Source: CAD feature listing. Evaluate the final solid. Frame: model axes, mm. Give positions to 0.01 mm unless a question says otherwise; leave off trailing zeros. Write each loop counter-clockwise with the first axis right and the second up, starting at its lowest first coordinate (ties: lowest second). Pieces come first, ordered by that corner, then holes. Notation, with made-up numbers: (82.5, 43) - (113.5, 43) arc R23 cw to (113.5, 81) - close; hole circle Ø3 at (35.5, -29.75). An arc over 180 degrees is marked (long way). One line per question, with ' | ' between items. Start each with the question number.
(1) Section A-A, the plane z = 2.75. Return loops of the section in (x, y) (3 decimals).
(2) Section D-D, the plane y = 2.75. Return loops of the section in (x, z) (3 decimals), plus the area to 3 significant figures.
(3) Ray query, line 1 (Y direction, x = 1, z = 17.75) (3 decimals); line 2 (Z direction, x = 1.05, y = 14.25); line 3 (Y direction, x = 1.45, z = 2). Return the intervals inside material, ascending. Write a range as [from, to].
(4) Draft query along Z for faces 1 (the flat face through (1.6, 13, 10)), 2 (the cylindrical face through (0.81, 22.63, 16.25)), 3 (the flat face through (1, 13, 0)). Return one class per face: +Z half, -Z half, draft (parallel to the pull), parting line (faces both ways), or undercut.
(5) Section B-B, the plane x = 0.35. State how many separate pieces and enclosed holes the cut face has, plus the area to 3 significant figures.
Autodesk Inventor part; units mm, degrees
ref_plane "YZ Plane" through (0, 0, 0) normal (1, 0, 0) x (0, 1, 0)
ref_plane "XZ Plane" through (0, 0, 0) normal (0, 1, 0) x (-1, 0, 0)
ref_plane "XY Plane" through (0, 0, 0) normal (0, 0, 1) x (1, 0, 0)
sketch "Náčrt1" plane through (0, 0, 0) normal (1, 0, 0) x (0, 1, 0)
  line L0 (0, 0) -> (26, 0)
  line L1 (26, 0) -> (26, 20.3)
  line L2 (26, 20.3) -> (0, 20.3)
  line L3 (0, 20.3) -> (0, 0)
  dimension "d0" = 26
  dimension "d1" = 20.3
extrude "Vysunutí1" add sketch "Náčrt1" along normal blind 1.6
sketch "Náčrt2" plane through (1.6, 0, 0) normal (1, 0, 0) x (0, 0, -1)
  line L0 (0, 0) -> (0, 26)
  line L1 (-20.3, 0) -> (0, 0)
  circle A0 centre (-2.75, 23.25) radius 1.625
  circle A1 centre (-2.75, 2.75) radius 1.625
  circle A2 centre (-1.27, 16.81) radius 0.45
  circle A3 centre (-1.27, 14.27) radius 0.45
  circle A4 centre (-1.27, 11.73) radius 0.45
  circle A5 centre (-1.27, 9.19) radius 0.45
  circle A6 centre (-17.75, 23.25) radius 1.625
  circle A7 centre (-17.75, 2.75) radius 1.625
  dimension "d4" = 20.5
  dimension "d6" = 3.25
  dimension "d7" = 2.75
  dimension "d8" = 2.75
  dimension "d9" = 2.75
  dimension "d10" = 0.9
  dimension "d11" = 1.27
  dimension "d12" = 2.54
  dimension "d13" = 2.54
  dimension "d14" = 2.54
  dimension "d15" = 1.27
  dimension "d16" = 1.27
  dimension "d17" = 1.27
  dimension "d18" = 7.62
  dimension "d19" = 6.44
  dimension "d20" = 20.5
  dimension "d21" = 2.75
  dimension "d25" = 15
  dimension "d26" = 15
extrude "Vysunutí3" cut sketch "Náčrt2" against normal through all
sketch "Náčrt3" plane through (1.6, 0, 0) normal (1, 0, 0) x (0, 0, -1)
  circle A0 centre (-1.27, 11.73) radius 0.45
  circle A1 centre (-1.27, 16.81) radius 0.45
  circle A2 centre (-1.27, 14.27) radius 0.45
  circle A3 centre (-1.27, 9.19) radius 0.45
  line L0 (-2.27, 17.7223) -> (-0.27, 17.7223)
  line L1 (-0.27, 17.7223) -> (-0.27, 15.7223)
  line L2 (-0.27, 15.7223) -> (-2.27, 15.7223)
  line L3 (-2.27, 15.7223) -> (-2.27, 17.7223)
  circle A4 centre (-1.27, 14.27) radius 1
  circle A5 centre (-1.27, 11.73) radius 1
  circle A6 centre (-1.27, 9.19) radius 1
  dimension "d31" = 2
  dimension "d33" = 1
  dimension "d34" = 2
  dimension "d35" = 1.0877
  dimension "d36" = 2
extrude "Vysunutí4" add sketch "Náčrt3" along normal blind 0.001
sketch "Náčrt4" plane through (0, 0, 0) normal (-1, 0, 0) x (0, 0, 1)
  circle A0 centre (1.27, 11.73) radius 0.45
  circle A1 centre (1.27, 16.81) radius 0.45
  circle A2 centre (1.27, 14.27) radius 0.45
  circle A3 centre (1.27, 9.19) radius 0.45
  line L0 (2.27, 17.7223) -> (0.27, 17.7223)
  line L1 (2.27, 15.7223) -> (2.27, 17.7223)
  line L2 (0.27, 15.7223) -> (2.27, 15.7223)
  line L3 (0.27, 17.7223) -> (0.27, 15.7223)
  circle A4 centre (1.27, 14.27) radius 1
  circle A5 centre (1.27, 11.73) radius 1
  circle A6 centre (1.27, 9.19) radius 1
extrude "Vysunutí5" add sketch "Náčrt4" along normal blind 0.001
sketch "Náčrt5" plane through (1.6, 0, 0) normal (1, 0, 0) x (0, 0, -1)
  line L0 (-12.9507, 18.458) -> (-3.259, 18.458) construction
  line L1 (-3.259, 18.458) -> (-3.259, 7.2075) construction
  line L2 (-3.259, 7.2075) -> (-12.9507, 7.2075) construction
  line L3 (-12.9507, 7.2075) -> (-12.9507, 18.458) construction
sketch "Náčrt6" plane through (0, 0, 0) normal (-1, 0, 0) x (0, 0, 1)
  line L0 (2.7892, 18.5709) -> (6.1278, 18.5709) construction
  line L1 (6.1278, 18.5709) -> (6.1278, 7.3401) construction
  line L2 (6.1278, 7.3401) -> (2.7892, 7.3401) construction
  line L3 (2.7892, 7.3401) -> (2.7892, 18.5709) construction
  line L4 (9.218, 26) -> (9.218, 0) construction
  line L5 (9.218, 0) -> (6.7421, 0) construction
  line L6 (6.7421, 0) -> (6.7421, 26) construction
  line L7 (6.7421, 26) -> (9.218, 26) construction
  line L8 (18.8, 26) -> (18.8, 0) construction
  line L9 (18.8, 0) -> (16.2512, 0) construction
  line L10 (16.2512, 0) -> (16.2512, 26) construction
  line L11 (16.2512, 26) -> (18.8, 26) construction
equation "\"d7\" = -0.5 * d4 + 0.5 * d0"
equation "\"d8\" = d7"
equation "\"d9\" = d7"
equation "\"d15\" = d11"
equation "\"d16\" = d11"
equation "\"d17\" = d11"
equation "\"d19\" = -0.5 * d18 + 0.5 * d4"
equation "\"d20\" = d4"
equation "\"d21\" = d7"
equation "\"d26\" = d25"
equation "\"PoloměrOhybu\" = Tloušťka"
equation "\"ŠířkaVýštipu\" = Tloušťka"
equation "\"HloubkaVýštipu\" = 0.5 * Tloušťka"
equation "\"VelikostRohovéhoVýštipu\" = 4 * Tloušťka"
equation "\"MinimálníZbytek\" = 2 * Tloušťka"
equation "\"PřechodovýPoloměr\" = PoloměrOhybu"
equation "\"VelikostJacobihoPoloměru\" = Tloušťka"
equation "\"VelikostMezery\" = Tloušťka"
properties part number "SparkFun USB Type A Female Breakout - doska" material "ABS plast"
Check sheet entries:
1) outline: (0, 0) - (1.6, 0) - (1.6, 1.125) - (0, 1.125) - close; (0, 4.375) - (1.6, 4.375) - (1.6, 21.625) - (0, 21.625) - close; (0, 24.875) - (1.6, 24.875) - (1.6, 26) - (0, 26) - close
2) outline: (0, 0) - (1.6, 0) - (1.6, 1.125) - (0, 1.125) - close; (0, 4.375) - (1.6, 4.375) - (1.6, 16.125) - (0, 16.125) - close; (0, 19.375) - (1.6, 19.375) - (1.6, 20.3) - (0, 20.3) - close | area: 22.1 mm²
3) line 1: [0, 1.125], [4.375, 21.625], [24.875, 26] | line 2: [0, 0.82], [1.72, 20.3] | line 3: [0, 1.31], [4.19, 21.81], [24.69, 26]
4) face 1: draft | face 2: undercut | face 3: -Z half
5) separate pieces: 1 | enclosed holes: 8 | area: 492 mm²
